Here's how the part is built. I have some questions about the finished solid (model axes, mm). A direction names the side the tool comes from. Coordinates: 2 decimals unless noted, no trailing zeros. Write each loop counter-clockwise with the first axis right and the second up, starting at its lowest first coordinate (ties: lowest second). Pieces come first, ordered by that corner, then holes.
(1) Which directions (+Z, -Z, +X, -X, +Y, -Y) give clear straight access to the entire face, cutting with the end or side of a thin tool? Please do faces 1 (the flat face through (-38, 55.253, 2)), 2 (the flat face through (-39, 51, 6)), 3 (the flat face through (-35.6, 48.753, 1.6)).
(2) Imagine slicing it at D-D, the plane x = -35.75. List the corners of the cut face in (y, z) for me.
(3) For pin 1 Ø3 at (y, z) = (46, 1) entering from -X; pin 2 Ø3 at (x, y) = (-43, 48.5) entering from -Z; pin 3 Ø1.8 at (x, z) = (-36, 1.5) entering from +Y; pin 4 Ø3 at (x, z) = (-38.5, 3) entering from -Y, each with a flat end and sliding along its axis, tell me the tip position at first contact or that it passes through.
(4) Imagine slicing it at A-A, the plane y = 46.25. List the corners of the cut face in (x, z) for me, plus the area to 3 significant figures.
(5) Imagine slicing it at C-C, the plane z = 3.35. List the corners of the cut face in (x, y) for me, plus the area to 3 significant figures.
(6) Please list where these lines run through material, in increasing order: probe 1 along X at (y, z) = (52.5, 3.3); probe 2 along X at (y, z) = (45.25, 2.2); probe 3 along Y at (x, z) = (-35, 1.15).
(7) Thinking about a two-plate mould opening in X: for faces 4 (the flat face through (-38, 43.253, 2)), 5 (the cylindrical face through (-35.05, 46.04, 3.03)), 6 (the flat face through (-32.823, 46, 3)), which applies, released by +X, released by -X, zero draft, split by the parting line, or undercut?
(8) Imagine slicing it at B-B, the plane x = -39.25. List the corners of the cut face in (y, z) for me.
```python
from build123d import *

# Parameters (mm, degrees)
BOSS_EXTRUDE1_DEPTH = 6
SKETCH2_R           = 1.5
CUT_EXTRUDE1_DEPTH  = 14


with BuildPart() as part:
    # Sketch1 → Boss-Extrude1 (new body)
    with BuildSketch(Plane.XY):
        with BuildLine():
            Line((-32.822846092, 55.253207469), (-40.85246604, 55.253207469))
            ThreePointArc((-40.85246604, 55.253207469), (-53.910402863, 49.253207469), (-40.85246604, 43.253207469))
            Line((-40.85246604, 43.253207469), (-32.822846092, 43.253207469))
            Line((-32.822846092, 43.253207469), (-32.822846092, 48.753207469))
            Line((-32.822846092, 48.753207469), (-38.111345814, 48.753207469))
            Line((-38.111345814, 48.753207469), (-40.124187091, 48.753207469))
            ThreePointArc((-40.124187091, 48.753207469), (-51.902962473, 49.253207469), (-40.124187091, 49.753207469))
            Line((-40.124187091, 49.753207469), (-38.111345814, 49.753207469))
            Line((-38.111345814, 49.753207469), (-32.822846092, 49.753207469))
            Line((-32.822846092, 49.753207469), (-32.822846092, 55.253207469))
        make_face()
    extrude(amount=BOSS_EXTRUDE1_DEPTH)

    # Sketch2 → Cut-Extrude1 (cut)
    with BuildSketch(Plane(origin=(0, 55.253207469, 0), x_dir=(1, 0, 0), z_dir=(0, 1, 0))):
        with Locations(Location((-36.547451728, -2.96481335, 0), (0, 0, 180))):
            Circle(SKETCH2_R)
    extrude(amount=-CUT_EXTRUDE1_DEPTH, mode=Mode.SUBTRACT)


solid = part.part
```
Recorded:
1. face 1: +Z, -Z, +X, +Y
1. face 2: +Z, +X, -X, +Y, -Y
1. face 3: +Z, -Z, +X
2. outline: (43.25, 0) - (48.75, 0) - (48.75, 1.69) - (43.25, 1.69) - close; (43.25, 4.24) - (48.75, 4.24) - (48.75, 6) - (43.25, 6) - close; (49.75, 0) - (55.25, 0) - (55.25, 1.69) - (49.75, 1.69) - close; (49.75, 4.24) - (55.25, 4.24) - (55.25, 6) - (49.75, 6) - close
3. pin 1: stops at x = -53.71
3. pin 2: passes through
3. pin 3: stops at y = 55.25
3. pin 4: stops at y = 43.25
4. outline: (-53.32, 0) - (-51.08, 0) - (-51.08, 6) - (-53.32, 6) - close; (-40.92, 0) - (-32.82, 0) - (-32.82, 6) - (-40.92, 6) - close; hole circle Ø3 at (-36.55, 2.96)
4. area: 55.0 mm2
5. outline: (-40.85, 43.25) - (-38, 43.25) - (-38, 48.75) - (-40.12, 48.75) arc R5.9 cw (long way) to (-40.12, 49.75) - (-38, 49.75) - (-38, 55.25) - (-40.85, 55.25) arc R7.91 ccw (long way) to start; (-35.1, 43.25) - (-32.82, 43.25) - (-32.82, 48.75) - (-35.1, 48.75) - close; (-35.1, 49.75) - (-32.82, 49.75) - (-32.82, 55.25) - (-35.1, 55.25) - close
5. area: 121 mm2
6. probe 1: x = -53.21 to -50.93, -41.08 to -38.01, -35.09 to -32.82
6. probe 2: x = -52.82 to -50.34, -41.67 to -37.84, -35.26 to -32.82
6. probe 3: y = 43.25 to 48.75, 49.75 to 55.25
7. face 4: zero draft
7. face 5: undercut
7. face 6: released by +X
8. outline: (43.25, 0) - (48.75, 0) - (48.75, 6) - (43.25, 6) - close; (49.75, 0) - (55.25, 0) - (55.25, 6) - (49.75, 6) - close
